```python
from build123d import *

# Parameters (mm, degrees)
F0_W     = 80
F0_H     = 20
F0_R     = 3
F0_R_2   = 2.75
F1_DEPTH = 8.5
F2_R     = 4.75
F2_R_2   = 2.75
F3_DEPTH = 6.5


with BuildPart() as f1:
    # F0 (on Front) → F1 (new body)
    with BuildSketch(Plane.XZ):
        with Locations((40, 10)):
            Rectangle(F0_W, F0_H)
        with Locations((40, 4.75)):
            Circle(F0_R, mode=Mode.SUBTRACT)
        with Locations((15, 14)):
            Circle(F0_R_2, mode=Mode.SUBTRACT)
        with Locations((65, 14)):
            Circle(F0_R_2, mode=Mode.SUBTRACT)
    extrude(amount=F1_DEPTH)

    # F2 (on face) → F3 (cut)
    with BuildSketch(Plane.XZ.offset(8.5)):
        with Locations((15, 14)):
            Circle(F2_R)
        with Locations((15, 14)):
            Circle(F2_R_2, mode=Mode.SUBTRACT)
        with Locations((65, 14)):
            Circle(F2_R)
        with Locations((65, 14)):
            Circle(F2_R_2, mode=Mode.SUBTRACT)
    extrude(amount=-F3_DEPTH, mode=Mode.SUBTRACT)


solid = f1.part
```
CAD build for the part. Positions are in the model's coordinates, mm. A direction names the side the tool comes from. Round coordinates to 2 decimals unless told otherwise and drop trailing zeros. Loops run counter-clockwise (first coordinate to the right, second up) from the corner with the lowest first, then second, coordinate; pieces in that order, holes last. Notation, with made-up numbers: M 13.25,47 L 36.25,47 A31 ccw 36.25,72 Z; hole C -29.5,48 d1. An arc over 180 degrees is marked long. Return JSON: item names as keys, results as strings. Group by question number.
(1) Tool access for faces 1 (the cylindrical face through (12.973, -0.986, 15.859)), 2 (the flat face through (68, -2, 14)): list every direction of +Z, -Z, +X, -X, +Y, -Y with a clear straight run to the whole face (end or side of a thin tool).
(2) Saw through at A-A, the plane z = 4.75. List the corners of the cut face in (x, y), and give its area (3 significant figures).
(3) Wall check: probe 1 along Z at (x, y) = (40, -3.25); probe 2 along Z at (x, y) = (65, -1.4); probe 3 along X at (y, z) = (-3, 16.75). Give the ranges that are in metal, low to high. Write a range as [from, to].
(4) Drop flat-ended pins along their axis: P1, Ø3, axis at x = 12.5, z = 15, coming from the -Y side; P2, Ø4, axis at x = 22, z = 8, coming from the +Y side; P3, Ø3.5, axis at x = 40, z = 4.75, coming from the +Y side. Give the stop position or say it passes through.
(5) Saw through at C-C, the plane y = -1. List the corners of the cut face in (x, z).
(6) Saw through at B-B, the plane x = 15. List the corners of the cut face in (y, z), and give its area (4 significant figures).
(7) Mould opens along X. For faces 3 (the flat face through (39, -8.5, 10)), 4 (the flat face through (80, -4, 10)), 5 (the flat face through (0, -4, 10)), 6 (the cylindrical face through (62.253, -0.986, 14.121)) say: +X half, -X half, draft (parallel to the pull), parting line (faces both ways), or undercut.
Answer list:
{
 "1": {"face 1": "+Y, -Y", "face 2": "-Y"},
 "2": {"outline": "M 0,-8.5 L 37,-8.5 L 37,0 L 0,0 Z; M 43,-8.5 L 80,-8.5 L 80,0 L 43,0 Z", "area": "629 mm2"},
 "3": {"probe 1": "[0, 1.75], [7.75, 20]", "probe 2": "[0, 11.25], [16.75, 20]", "probe 3": "[0, 11.13], [18.87, 61.13], [68.87, 80]"},
 "4": {"P1": "y = -2", "P2": "y = 0", "P3": "through"},
 "5": {"outline": "M 0,0 L 80,0 L 80,20 L 0,20 Z; hole C 15,14 d5.5; hole C 40,4.75 d6; hole C 65,14 d5.5"},
 "6": {"outline": "M -8.5,0 L 0,0 L 0,11.25 L -2,11.25 L -2,9.25 L -8.5,9.25 Z; M -8.5,18.75 L -2,18.75 L -2,16.75 L 0,16.75 L 0,20 L -8.5,20 Z", "area": "97.25 mm2"},
 "7": {"face 3": "draft", "face 4": "+X half", "face 5": "-X half", "face 6": "undercut"}
}
